```python
from build123d import *

# Parameters (mm, degrees)
SKETCH1_R           = 2.5
BOSS_EXTRUDE1_DEPTH = 16
SKETCH2_R           = 3.5
BOSS_EXTRUDE2_DEPTH = 4
CHAMFER1_SIZE       = 1
CUT_EXTRUDE1_DEPTH  = 3


with BuildPart() as part:
    # Sketch1 → Boss-Extrude1 (new body)
    with BuildSketch(Plane(origin=(0, 0, 0), x_dir=(1, 0, 0), z_dir=(0, 1, 0))):
        with Locations(Location((0, 0, 0), (0, 0, 270))):
            Circle(SKETCH1_R)
    extrude(amount=BOSS_EXTRUDE1_DEPTH)

    # Sketch2 → Boss-Extrude2 (add)
    with BuildSketch(Plane(origin=(0, 16, 0), x_dir=(1, 0, 0), z_dir=(0, 1, 0))):
        with Locations(Location((0, 0, 0), (0, 0, 270))):
            Circle(SKETCH2_R)
    extrude(amount=BOSS_EXTRUDE2_DEPTH)

    # Chamfer1
    chamfer1_edges = [part.edges().sort_by_distance(p)[0] for p in [
        (0, 0, -2.5),
    ]]
    chamfer(chamfer1_edges, length=CHAMFER1_SIZE)

    # Sketch3 → Cut-Extrude1 (cut)
    with BuildSketch(Plane(origin=(0, 20, 0), x_dir=(1, 0, 0), z_dir=(0, 1, 0))):
        Polygon((2.309401077, 0), (1.154700538, 2), (-1.154700538, 2), (-2.309401077, 0), (-1.154700538, -2), (1.154700538, -2), align=None)
    extrude(amount=-CUT_EXTRUDE1_DEPTH, mode=Mode.SUBTRACT)


solid = part.part
```
Verification items for the finished model (mm, model axes). A direction names the side the tool comes from. Round coordinates to 2 decimals unless told otherwise and drop trailing zeros. Loops run counter-clockwise (first coordinate to the right, second up) from the corner with the lowest first, then second, coordinate; pieces in that order, holes last. Notation, with made-up numbers: (8, 57.5) -> (51, 57.5) arc R27 cw to (51, 79.5) -> close; hole circle Ø7 at (52.5, -33.5). An arc over 180 degrees is marked (long way). Answer as a JSON object with one key per item and string values.
Q1. Draft check along X on faces 1 (the cylindrical face through (-3.417, 17.972, -0.759)), 2 (the flat face through (0, 17, 0)), 3 (the flat face through (0, 0, 0)). Enter one of: pulls with the +X half, pulls with the -X half, needs draft (parallel to the pull), parting line crosses it, or undercut.
Data:
{"face 1": "parting line crosses it", "face 2": "undercut", "face 3": "needs draft"}
Q2. Scan lines: line 1 (Y direction, x = -0.25, z = 3.25); line 2 (Y direction, x = 0.5, z = 0); line 3 (Z direction, x = -1.5, y = 17.25). Record each from-to range of solid material in increasing order. Write a range as from..to.
Data:
{"line 1": "y = 16..20", "line 2": "y = 0..17", "line 3": "z = -3.16..-1.4, 1.4..3.16"}
Q3. Section check A-A (x = 0). Record the boundary of the cut face in (y, z), then the cut area to 3 significant figures.
Data:
{"outline": "(0, -1.5) -> (1, -2.5) -> (16, -2.5) -> (16, -3.5) -> (20, -3.5) -> (20, -2) -> (17, -2) -> (17, 2) -> (20, 2) -> (20, 3.5) -> (16, 3.5) -> (16, 2.5) -> (1, 2.5) -> (0, 1.5) -> close", "area": "95.0 mm2"}
Q4. Section check D-D (x = -3). Record the boundary of the cut face in (y, z).
Data:
{"outline": "(16, -1.8) -> (20, -1.8) -> (20, 1.8) -> (16, 1.8) -> close"}
Q5. Go/stop test with flat-tipped pins: P1, Ø2, axis at x = -0.5, z = 1, coming from the -Y side; P2, Ø2, axis at y = 4, z = 0.5, coming from the -X side; P3, Ø1, axis at x = -1.5, y = 9.5, coming from the +Z side. Record where each tip stops, or that it passes through.
Data:
{"P1": "stops at y = 0", "P2": "stops at x = -2.5", "P3": "stops at z = 2.29"}
Q6. Access from +Z, -Z, +X, -X, +Y, -Y to the whole of each face (thin tool, end or side, straight path). Record for faces 4 (the cylindrical face through (-2.44, 8.4, -0.54)), 5 (the flat face through (0, 19, 2)), 6 (the flat face through (-2, 20, 2)).
Data:
{"face 4": "-Y", "face 5": "+Y", "face 6": "+Z, -Z, +X, -X, +Y"}
Q7. Section check B-B (y = 4.25). Record the boundary of the cut face in (x, z), then the cut area to 3 significant figures.
Data:
{"outline": "circle Ø5 at (0, 0)", "area": "19.6 mm2"}
Q8. Section check C-C (z = -3). Record the boundary of the cut face in (x, y).
Data:
{"outline": "(-1.8, 16) -> (1.8, 16) -> (1.8, 20) -> (-1.8, 20) -> close"}
